The listing builds one solid part. Answer for the finished solid, in the listing's coordinates (mm). A direction names the side the tool comes from. Coordinates: 2 decimals unless noted, no trailing zeros. Write each loop counter-clockwise with the first axis right and the second up, starting at its lowest first coordinate (ties: lowest second). Pieces come first, ordered by that corner, then holes.
(1) The part is cut by section B-B on z = 0. Determine the outline of the cut face in (x, y), plus the area to 3 significant figures.
(2) Which of the six approach directions +Z, -Z, +X, -X, +Y, -Y give full straight-line access (tool end or side, diameter ignored) to faces 5 (the flat face through (8, -5, -1.984)), 6 (the flat face through (0, -6.35, 5))?
(3) Straight lines are drawn through the part: line 1 (Z direction, x = 0, y = -1.75); line 2 (Z direction, x = -2, y = -3.25). For each, find the intervals that lie inside material, in ascending order.
(4) For a pull along Z with two mould halves and no side action, classify faces 1 (the cylindrical face through (-1.55, -2.425, 11.805)), 2 (the flat face through (-8, -5, -1.984)), 3 (the flat face through (0, -3.175, -7)), 4 (the cylindrical face through (2.56, -3.219, 4.016)) as +Z half, -Z half, draft (parallel to the pull), parting line (faces both ways), or undercut.
(5) The part is cut by section D-D on y = -5.25. Determine the outline of the cut face in (x, z) (1 decimal).
(6) The part is cut by section C-C on y = -1. Determine the outline of the cut face in (x, z) (1 decimal).
(7) Given P1, Ø1.5, axis at x = -4.5, y = -1, coming from the +Z side; P2, Ø1.5, axis at y = -1.5, z = 5.5, coming from the -X side; P3, Ø1, axis at x = -6.5, y = -4.5, coming from the -Z side; P4, Ø10, axis at x = 0, z = 6, coming from the +Y side, each flat-ended and moving along its own axis, determine where each tip first touches the part or whether it passes through.
from build123d import *

# Parameters (mm, degrees)
F0_R     = 11.90625
F1_DEPTH = 6.35
F2_R     = 4.7625
F3_DEPTH = 25.4
F5_DEPTH = 3.175


with BuildPart() as f1:
    # F0 (on Front) → F1 (new body)
    with BuildSketch(Plane.XZ):
        Circle(F0_R)
    extrude(amount=F1_DEPTH)

    # F2 (on face) → F3 (cut)
    with BuildSketch(Plane.XZ.offset(6.35)):
        Circle(F2_R)
    extrude(amount=-F3_DEPTH, mode=Mode.SUBTRACT)

    # F4 (on face) → F5 (cut)
    with BuildSketch(Plane.XZ.offset(6.35)):
        with BuildLine():
            Line((-4.329395, -1.984375), (-11.739721, -1.984375))
            ThreePointArc((-11.739721, -1.984375), (0, -11.90625), (11.739721, -1.984375))
            Line((11.739721, -1.984375), (4.329395, -1.984375))
            ThreePointArc((4.329395, -1.984375), (0, -4.7625), (-4.329395, -1.984375))
        make_face()
        with BuildLine():
            Line((4.329395, -1.984375), (-4.329395, -1.984375))
            ThreePointArc((-4.329395, -1.984375), (0, -4.7625), (4.329395, -1.984375))
        make_face()
    extrude(amount=-F5_DEPTH, mode=Mode.SUBTRACT)


solid = f1.part
Model answer:
1. outline: (-11.91, -6.35) - (-4.76, -6.35) - (-4.76, 0) - (-11.91, 0) - close; (4.76, -6.35) - (11.91, -6.35) - (11.91, 0) - (4.76, 0) - close
1. area: 90.7 mm2
2. face 5: -Z, +X, -X, -Y
2. face 6: +Z, -Z, +X, -X, -Y
3. line 1: z = -11.91 to -4.76, 4.76 to 11.91
3. line 2: z = 4.32 to 11.74
4. face 1: parting line
4. face 2: -Z half
4. face 3: draft
4. face 4: undercut
5. outline: (-11.7, -2) - (-4.3, -2) arc R4.8 cw (long way) to (4.3, -2) - (11.7, -2) arc R11.9 ccw (long way) to start
6. outline: circle Ø23.8 at (0, 0); hole circle Ø9.5 at (0, 0)
7. P1: stops at z = 11.3
7. P2: stops at x = -10.92
7. P3: stops at z = -1.98
7. P4: stops at y = 0
